Check sheet for the modelled part. Datum: model origin and axes. Units: mm. A direction names the side the tool comes from. Give positions to 0.01 mm unless a question says otherwise; leave off trailing zeros. Write each loop counter-clockwise with the first axis right and the second up, starting at its lowest first coordinate (ties: lowest second). Pieces come first, ordered by that corner, then holes. Notation, with made-up numbers: M 65.25,66.5 L 89.25,66.5 A28 cw 89.25,97.5 Z; hole C 40.5,51 d8. An arc over 180 degrees is marked long. Write item = value, one per line. Start each with the question number.
1) Set-up check for faces 4 (the face through (12, 22, -6)), 5 (the face through (13, 22, 1.75)), 6 (the face through (1, 42.2, 3)), 7 (the face through (0.121, 5.373, -19.247)), 8 (the face through (-4, 7, -17)): record each of +Z, -Z, +X, -X, +Y, -Y from which the full face is reachable in a straight line by a thin tool's end or side.
2) Draft check along X on faces 1 (the face through (6.5, 40, -1.4)), 2 (the face through (-6.5, 4.1, -1.4)), 3 (the face through (0, 3, -20.5)). Enter one of: pulls with the +X half, pulls with the -X half, needs draft (parallel to the pull), parting line crosses it, or undercut.
3) Sectioned sample at C-C, the plane x = 13. Record the cut outline in (y, z).
4) Scan lines: L1, parallel to X at y = 43, z = 0; L2, parallel to X at y = 15, z = 5; L3, parallel to Y at x = 10, z = -4.5. Record each from-to range of solid material in increasing order.
5) Sectioned sample at B-B, the plane y = 18. Record the cut outline in (x, z), then the cut area to 4 significant figures.
6) Sectioned sample at A-A, the plane z = -16.5. Record the cut outline in (x, y).
7) Sectioned sample at D-D, the plane y = 4.5. Record the cut outline in (x, z).
8) Gauge pin test, flat ends, axial feed: pin 1 (2.5 mm diameter, centred on x = 13.5, y = 19, fed in from -Z); pin 2 (3 mm diameter, centred on x = 0, z = 16.5, fed in from -Y); pin 3 (6 mm diameter, centred on x = -1, z = 16, fed in from +Y); pin 4 (0.9 mm diameter, centred on x = 14, y = 20.5, fed in from +Z). Record the tip position at first contact, or that the pin passes through.
from build123d import *

# Parameters (mm, degrees)
SKETCH1_W               = 30
SKETCH1_H               = 25
BOSS_EXTRUDE1_DEPTH     = 7
BOSS_EXTRUDE2_DEPTH     = 30
SKETCH3_W               = 30
SKETCH3_H               = 25
BOSS_EXTRUDE3_DEPTH     = 7
SKETCH4_R               = 7.65
CUT_EXTRUDE1_DEPTH      = 1.3
CUT_EXTRUDE2_START      = -1.3
SKETCH5_R               = 7.65
CUT_EXTRUDE2_DEPTH      = 1.3
SKETCH6_R               = 6.65
CUT_EXTRUDE3_DEPTH      = 3.3
CUT_EXTRUDE4_START      = -3.3
SKETCH7_R               = 6.65
CUT_EXTRUDE4_DEPTH      = 3.3
SKETCH8_R               = 4.75
CUT_EXTRUDE5_DEPTH      = 0.6
CUT_EXTRUDE6_START      = -0.6
SKETCH9_R               = 4.75
CUT_EXTRUDE6_DEPTH      = 0.6
CUT_EXTRUDE7_DEPTH      = 47.498279538
CUT_EXTRUDE7_DEPTH_BACK = 47.498279538
SKETCH10_R              = 3
CUT_EXTRUDE8_DEPTH      = 55.701462503
CUT_EXTRUDE8_DEPTH_BACK = 10.6
SKETCH11_W              = 3.5
SKETCH11_H              = 30
SKETCH12_W              = 30
SKETCH12_H              = 8
SKETCH12_R              = 1.65
BOSS_EXTRUDE4_DEPTH     = 7
SKETCH13_R              = 2.75
CUT_EXTRUDE9_DEPTH      = 3.3


with BuildPart() as part:
    # Sketch1 → Boss-Extrude1 (new body)
    with BuildSketch(Plane(origin=(0, 0, 0), x_dir=(1, 0, 0), z_dir=(0, 1, 0))):
        Rectangle(SKETCH1_W, SKETCH1_H)
    extrude(amount=BOSS_EXTRUDE1_DEPTH)

    # Sketch2 → Boss-Extrude2 (add)
    with BuildSketch(Plane(origin=(0, 7, 0), x_dir=(1, 0, 0), z_dir=(0, 1, 0))):
        Polygon((-15, -12.5), (-12, -12.5), (-12, 9.5), (12, 9.5), (12, -12.5), (15, -12.5), (15, 12.5), (-15, 12.5), align=None)
    extrude(amount=BOSS_EXTRUDE2_DEPTH)

    # Sketch3 → Boss-Extrude3 (add)
    with BuildSketch(Plane(origin=(0, 37, 0), x_dir=(1, 0, 0), z_dir=(0, 1, 0))):
        Rectangle(SKETCH3_W, SKETCH3_H)
    extrude(amount=BOSS_EXTRUDE3_DEPTH)

    # Sketch4 → Cut-Extrude1 (cut)
    with BuildSketch(Plane(origin=(0, 7, 0), x_dir=(1, 0, 0), z_dir=(0, 1, 0))):
        with Locations(Location((0, 0, 0), (0, 0, 270))):
            Circle(SKETCH4_R)
    extrude(amount=-CUT_EXTRUDE1_DEPTH, mode=Mode.SUBTRACT)

    # Sketch5 → Cut-Extrude2 (cut)
    with BuildSketch(Plane.XZ.offset(-37).offset(CUT_EXTRUDE2_START)):
        with Locations(Location((0, 0, 0), (0, 0, 90))):
            Circle(SKETCH5_R)
    extrude(amount=CUT_EXTRUDE2_DEPTH, mode=Mode.SUBTRACT)

    # Sketch6 → Cut-Extrude3 (cut)
    with BuildSketch(Plane(origin=(0, 5.7, 0), x_dir=(1, 0, 0), z_dir=(0, 1, 0))):
        with Locations(Location((0, 0, 0), (0, 0, 270))):
            Circle(SKETCH6_R)
    extrude(amount=-CUT_EXTRUDE3_DEPTH, mode=Mode.SUBTRACT)

    # Sketch7 → Cut-Extrude4 (cut)
    with BuildSketch(Plane.XZ.offset(-38.3).offset(CUT_EXTRUDE4_START)):
        with Locations(Location((0, 0, 0), (0, 0, 90))):
            Circle(SKETCH7_R)
    extrude(amount=CUT_EXTRUDE4_DEPTH, mode=Mode.SUBTRACT)

    # Sketch8 → Cut-Extrude5 (cut)
    with BuildSketch(Plane(origin=(0, 2.4, 0), x_dir=(1, 0, 0), z_dir=(0, 1, 0))):
        with Locations(Location((0, 0, 0), (0, 0, 270))):
            Circle(SKETCH8_R)
    extrude(amount=-CUT_EXTRUDE5_DEPTH, mode=Mode.SUBTRACT)

    # Sketch9 → Cut-Extrude6 (cut)
    with BuildSketch(Plane.XZ.offset(-41.6).offset(CUT_EXTRUDE6_START)):
        with Locations(Location((0, 0, 0), (0, 0, 90))):
            Circle(SKETCH9_R)
    extrude(amount=CUT_EXTRUDE6_DEPTH, mode=Mode.SUBTRACT)

    # Sketch10 → Cut-Extrude7 (cut, two sides: drawn at the far end of the back side and taken through both)
    with BuildSketch(Plane(origin=(0, 1.8, 0), x_dir=(1, 0, 0), z_dir=(0, 1, 0)).offset(-CUT_EXTRUDE7_DEPTH_BACK)):
        with Locations(Location((0, 0, 0), (0, 0, 270))):
            Circle(SKETCH10_R)
    extrude(amount=CUT_EXTRUDE7_DEPTH + CUT_EXTRUDE7_DEPTH_BACK, mode=Mode.SUBTRACT)

    # Sketch11 → Cut-Extrude8 (cut, two sides: drawn at the far end of the back side and taken through both)
    with BuildSketch(Plane(origin=(15, 0, 0), x_dir=(0, 0, -1), z_dir=(1, 0, 0)).offset(-CUT_EXTRUDE8_DEPTH_BACK)):
        with Locations((0, 22)):
            Rectangle(SKETCH11_W, SKETCH11_H)
    extrude(amount=CUT_EXTRUDE8_DEPTH + CUT_EXTRUDE8_DEPTH_BACK, mode=Mode.SUBTRACT)

    # Sketch12 → Boss-Extrude4 (add)
    # profile 1 of 2: a face of its own
    with BuildSketch(Plane(origin=(0, 0, 0), x_dir=(1, 0, 0), z_dir=(0, 1, 0))):
        with Locations((0, -16.5)):
            Rectangle(SKETCH12_W, SKETCH12_H)
        with Locations(Location((0, -16.5, 0), (0, 0, 270))):
            Circle(SKETCH12_R, mode=Mode.SUBTRACT)
    # profile 2 of 2: a face of its own
    with BuildSketch(Plane(origin=(0, 0, 0), x_dir=(1, 0, 0), z_dir=(0, 1, 0))):
        with Locations((0, 16.5)):
            Rectangle(SKETCH12_W, SKETCH12_H)
        with Locations(Location((0, 16.5, 0), (0, 0, 90))):
            Circle(SKETCH12_R, mode=Mode.SUBTRACT)
    extrude(amount=BOSS_EXTRUDE4_DEPTH)

    # Sketch13 → Cut-Extrude9 (cut)
    with BuildSketch(Plane(origin=(0, 7, 0), x_dir=(1, 0, 0), z_dir=(0, 1, 0))):
        with Locations(Location((0, 16.5, 0), (0, 0, 270))):
            Circle(SKETCH13_R)
        with Locations(Location((0, -16.5, 0), (0, 0, 270))):
            Circle(SKETCH13_R)
    extrude(amount=-CUT_EXTRUDE9_DEPTH, mode=Mode.SUBTRACT)


solid = part.part
Data:
q1.face_4 = +Z
q1.face_5 = +X
q1.face_6 = none
q1.face_7 = +Y
q1.face_8 = -Z, +X, -X, +Y
q2.face_1 = undercut
q2.face_2 = undercut
q2.face_3 = needs draft
q3.outline = M 0,-20.5 L 7,-20.5 L 7,-12.5 L 44,-12.5 L 44,12.5 L 7,12.5 L 7,20.5 L 0,20.5 Z; hole M 7,-1.75 L 37,-1.75 L 37,1.75 L 7,1.75 Z
q4.L1 = -15 to -3, 3 to 15
q4.L2 = -15 to -12, 12 to 15
q4.L3 = 0 to 7, 37 to 44
q5.outline = M -15,-12.5 L 15,-12.5 L 15,-1.75 L 12,-1.75 L 12,-9.5 L -12,-9.5 L -12,12.5 L -15,12.5 Z; M 12,1.75 L 15,1.75 L 15,12.5 L 12,12.5 Z
q5.area = 211.5 mm2
q6.outline = M -15,0 L -1.65,0 L -1.65,3.7 L -2.75,3.7 L -2.75,7 L -15,7 Z; M 1.65,0 L 15,0 L 15,7 L 2.75,7 L 2.75,3.7 L 1.65,3.7 Z
q7.outline = M -15,-20.5 L 15,-20.5 L 15,20.5 L -15,20.5 Z; hole C 0,0 d13.3; hole C 0,-16.5 d5.5; hole C 0,16.5 d5.5
q8.pin_1 = -12.5
q8.pin_2 = through
q8.pin_3 = 7
q8.pin_4 = 12.5
